```python
from build123d import *

# Parameters (mm, degrees)
SKETCH1_W               = 12.7
SKETCH1_H               = 12.7
SKETCH1_W_2             = 9.525
SKETCH1_H_2             = 9.525
BOSS_EXTRUDE1_DEPTH     = 185.42
CUT_EXTRUDE1_DEPTH      = 186.637338378
CUT_EXTRUDE1_DEPTH_BACK = 186.637338378
CUT_EXTRUDE2_DEPTH      = 186.637338378
CUT_EXTRUDE2_DEPTH_BACK = 186.637338378


with BuildPart() as part:
    # Sketch1 → Boss-Extrude1 (new, symmetric)
    with BuildSketch(Plane(origin=(0, 0, 0), x_dir=(0, 0, -1), z_dir=(1, 0, 0))):
        Rectangle(SKETCH1_W, SKETCH1_H)
        Rectangle(SKETCH1_W_2, SKETCH1_H_2, mode=Mode.SUBTRACT)
    extrude(amount=BOSS_EXTRUDE1_DEPTH, both=True)

    # Sketch2 → Cut-Extrude1 (cut, two sides: drawn at the far end of the back side and taken through both)
    with BuildSketch(Plane(origin=(0, 0, 0), x_dir=(1, 0, 0), z_dir=(0, 1, 0)).offset(-CUT_EXTRUDE1_DEPTH_BACK)):
        Polygon((-185.42, -6.35), (-174.250456919, 6.961343094), (-183.078216502, 14.368712905), (-194.247759583, 1.057369811), align=None)
    extrude(amount=CUT_EXTRUDE1_DEPTH + CUT_EXTRUDE1_DEPTH_BACK, mode=Mode.SUBTRACT)

    # Sketch3 → Cut-Extrude2 (cut, two sides: drawn at the far end of the back side and taken through both)
    with BuildSketch(Plane(origin=(0, 0, 0), x_dir=(1, 0, 0), z_dir=(0, 1, 0)).offset(-CUT_EXTRUDE2_DEPTH_BACK)):
        Polygon((185.42, 6.35), (173.150938826, -6.35), (185.42, -6.35), align=None)
    extrude(amount=CUT_EXTRUDE2_DEPTH + CUT_EXTRUDE2_DEPTH_BACK, mode=Mode.SUBTRACT)


solid = part.part
```
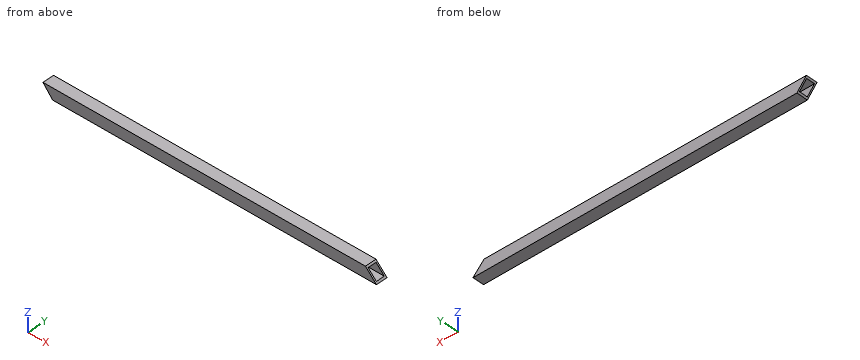
Can you work these out from the model? Positions are in its coordinate system, mm. Give positions to 0.01 mm unless a question says otherwise; leave off trailing zeros. Order: outer loops, then holes, each group sorted by start corner. A loop starts at its lowest first (then second) coordinate and runs counter-clockwise, first axis right, second up. Notation, with made-up numbers: M 43,6 L 68,6 A24 cw 68,26 Z; hole C -38,-20 d4. An arc over 180 degrees is marked long. Write item = value, one per line. Start each with the question number.
Q1. I need wall thicknesses on probe 1 along Y at (x, z) = (-65, 0). Which ranges of the line are inside material? Lowest first, please. Write a range as [from, to].
Q2. Suppose I cut it at B-B (z = -0.25). Write out the boundary of the cut face in (x, y), plus the area to 3 significant figures.
Q3. Suppose I cut it at A-A (x = 110). Write out the boundary of the cut face in (y, z).
Check result:
q1.probe_1 = [-6.35, -4.76], [4.76, 6.35]
q2.outline = M -179.88,-6.35 L 179.53,-6.35 L 179.53,-4.76 L -179.88,-4.76 Z; M -179.88,4.76 L 179.53,4.76 L 179.53,6.35 L -179.88,6.35 Z
q2.area = 1,140 mm2
q3.outline = M -6.35,-6.35 L 6.35,-6.35 L 6.35,6.35 L -6.35,6.35 Z; hole M -4.76,-4.76 L 4.76,-4.76 L 4.76,4.76 L -4.76,4.76 Z
